from build123d import *

# Parameters (mm, degrees)
BOSS_EXTRUDE2_DEPTH = 6.35
BOSS_EXTRUDE3_DEPTH = 6.35
SKETCH3_R           = 1.3716
CUT_EXTRUDE1_DEPTH  = 7.35
SKETCH4_R           = 6.35
CUT_EXTRUDE2_DEPTH  = 7.35
SKETCH5_R           = 1.905
CUT_EXTRUDE3_DEPTH  = 7.35
SKETCH7_R           = 1.85
CUT_EXTRUDE4_DEPTH  = 7.35


with BuildPart() as part:
    # Sketch1 → Boss-Extrude2 (new body)
    with BuildSketch(Plane(origin=(0, 0, 0), x_dir=(1, 0, 0), z_dir=(0, 1, 0))):
        Polygon((73.764977758, 99.321348004), (-18.071082704, 122.390514677), (-99.321348004, 73.764977758), (-122.390514677, -18.071082704), (-73.764977758, -99.321348004), (18.071082704, -122.390514677), (99.321348004, -73.764977758), (122.390514677, 18.071082704), align=None)
    extrude(amount=BOSS_EXTRUDE2_DEPTH)

    # Sketch2 → Boss-Extrude3 (add)
    with BuildSketch(Plane(origin=(0, 6.35, 0), x_dir=(-1, 0, 0), z_dir=(0, 1, 0))):
        Polygon((75.591082235, 96.270040344), (95.206631479, 108.009283415), (78.249947043, 136.342854545), (33.35213433, 109.473031516), (73.764977758, 99.321348004), align=None)
    extrude(amount=-BOSS_EXTRUDE3_DEPTH)

    # Sketch3 → Cut-Extrude1 (cut, through all)
    with BuildSketch(Plane.XZ):
        with Locations((-12.844640601, -78.437638464)):
            Circle(SKETCH3_R)
        with Locations((-35.416692023, -2.204063982)):
            Circle(SKETCH3_R)
        with Locations((-63.056087654, -48.387784923)):
            Circle(SKETCH3_R)
        with Locations((14.794755029, -32.253917523)):
            Circle(SKETCH3_R)
    extrude(amount=-CUT_EXTRUDE1_DEPTH, mode=Mode.SUBTRACT)

    # Sketch4 → Cut-Extrude2 (cut, through all)
    with BuildSketch(Plane.XZ):
        with Locations((-61.737440704, -17.814468138)):
            Circle(SKETCH4_R)
    extrude(amount=-CUT_EXTRUDE2_DEPTH, mode=Mode.SUBTRACT)

    # Sketch5 → Cut-Extrude3 (cut, through all)
    with BuildSketch(Plane.XZ):
        with Locations((2.267257691, -79.060054342)):
            Circle(SKETCH5_R)
        with Locations((-70.746175604, -35.363982912)):
            Circle(SKETCH5_R)
        with Locations((38.137167074, -19.123653876)):
            Circle(SKETCH5_R)
        with Locations((-34.876266221, 24.572417555)):
            Circle(SKETCH5_R)
    extrude(amount=-CUT_EXTRUDE3_DEPTH, mode=Mode.SUBTRACT)

    # Sketch7 → Cut-Extrude4 (cut, through all)
    with BuildSketch(Plane(origin=(0, 6.35, 0), x_dir=(1, 0, 0), z_dir=(0, 1, 0))):
        with Locations((15.538619902, -60.042079341)):
            Circle(SKETCH7_R)
        with Locations((-3.461904754, -28.29337759)):
            Circle(SKETCH7_R)
        with Locations((26.570650956, -10.319908322)):
            Circle(SKETCH7_R)
        with Locations((45.571175611, -42.068610072)):
            Circle(SKETCH7_R)
    extrude(amount=-CUT_EXTRUDE4_DEPTH, mode=Mode.SUBTRACT)


solid = part.part
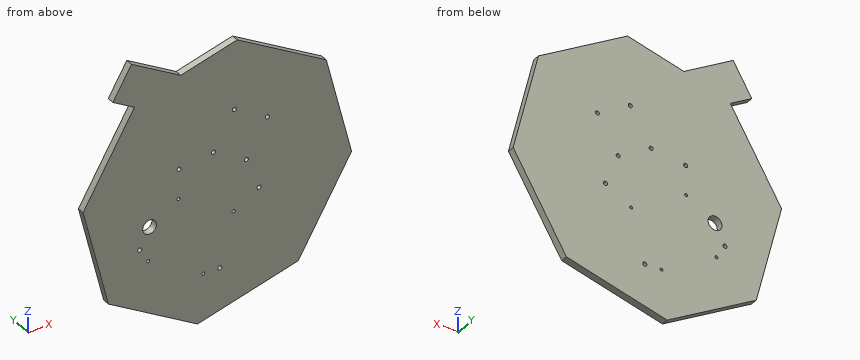
The listing builds one solid part. Answer for the finished solid, in the listing's coordinates (mm). Coordinates: 2 decimals unless noted, no trailing zeros. Write each loop counter-clockwise with the first axis right and the second up, starting at its lowest first coordinate (ties: lowest second). Pieces come first, ordered by that corner, then holes. Notation, with made-up numbers: (-32, 66) -> (3, 66) arc R13 cw to (3, 77) -> close; hole circle Ø2 at (30.25, 27.5). An arc over 180 degrees is marked (long way). One line per question, with ' | ' between items.
1. Section B-B (z = 88) is taken. Determine the outline of the cut face in (x, y), and give its area (3 significant figures).
Verdict:
outline: (-80.54, 0) -> (75.54, 0) -> (75.54, 6.35) -> (-80.54, 6.35) -> close | area: 991 mm^2
2. Section C-C (x = -105) is taken. Determine the outline of the cut face in (y, z), and give its area (3 significant figures).
Verdict:
outline: (0, -51.16) -> (6.35, -51.16) -> (6.35, 47.13) -> (0, 47.13) -> close | area: 624 mm^2
3. Section A-A (y = 3) is taken. State how many separate pieces and enclosed holes the cut face has, and give its area (3 significant figures).
Verdict:
separate pieces: 1 | enclosed holes: 13 | area: 44,200 mm^2
4. Straight lines are drawn through the part: line 1 (Z direction, x = 28, y = 0.5); line 2 (Z direction, x = -12, y = 4.5); line 3 (X direction, y = 4.5, z = -12.5). For each, find the intervals that lie inside material, in ascending order.
Verdict:
line 1: z = -110.82 to 9.15, 11.49 to 116.45 | line 2: z = -120.87 to -79.52, -77.36 to 114.84 | line 3: x = -114.71 to -65.21, -58.26 to 120.99
5. Given pin 1 Ø6 at (x, z) = (-70.75, -35.36) entering from -Y; pin 2 Ø1 at (y, z) = (4.5, 54.5) entering from +X; pin 3 Ø2 at (x, z) = (15.54, 60.04) entering from -Y; pin 4 Ø2 at (y, z) = (3, -57) entering from +X, each flat-ended and moving along its own axis, determine where each tip first touches the part or whether it passes through.
Verdict:
pin 1: stops at y = 0 | pin 2: stops at x = 104.29 | pin 3: passes through | pin 4: stops at x = 99.69
